from build123d import *

# Parameters (mm, degrees)
ESQUISSE1_R        = 1.5
BOSS_EXTRU_2_DEPTH = 6


with BuildPart() as part:
    # Esquisse1 → Boss.-Extru.2 (new body)
    with BuildSketch(Plane.XY):
        with BuildLine():
            Line((-4.997277712, 16.248914286), (-3.997277712, 21.633810827))
            ThreePointArc((-3.997277712, 21.633810827), (0.002768431, 21.999999826), (4.002722288, 21.632804124))
            Line((4.002722288, 21.632804124), (5.002722288, 16.247238834))
            ThreePointArc((5.002722288, 16.247238834), (8.502466554, 14.721007523), (11.573333699, 12.452226592))
            Line((11.573333699, 12.452226592), (16.7367909, 14.278649458))
            ThreePointArc((16.7367909, 14.278649458), (19.053942948, 10.997602381), (20.735919071, 7.349942877))
            Line((20.735919071, 7.349942877), (16.571882715, 3.791134828))
            ThreePointArc((16.571882715, 3.791134828), (16.999999761, -0.002848269), (16.570611412, -3.796687694))
            Line((16.570611412, -3.796687694), (20.734068613, -7.355161368))
            ThreePointArc((20.734068613, -7.355161368), (19.051174517, -11.002397445), (16.733196783, -14.282861248))
            Line((16.733196783, -14.282861248), (11.569160427, -12.456104006))
            ThreePointArc((11.569160427, -12.456104006), (8.497533208, -14.723855792), (4.997277712, -16.248914286))
            Line((4.997277712, -16.248914286), (3.997277712, -21.633810827))
            ThreePointArc((3.997277712, -21.633810827), (-0.002768431, -21.999999826), (-4.002722288, -21.632804124))
            Line((-4.002722288, -21.632804124), (-5.002722288, -16.247238834))
            ThreePointArc((-5.002722288, -16.247238834), (-8.502466554, -14.721007523), (-11.573333699, -12.452226592))
            Line((-11.573333699, -12.452226592), (-16.7367909, -14.278649458))
            ThreePointArc((-16.7367909, -14.278649458), (-19.053942948, -10.997602381), (-20.735919071, -7.349942877))
            Line((-20.735919071, -7.349942877), (-16.571882715, -3.791134828))
            ThreePointArc((-16.571882715, -3.791134828), (-16.999999761, 0.002848269), (-16.570611412, 3.796687694))
            Line((-16.570611412, 3.796687694), (-20.734068613, 7.355161368))
            ThreePointArc((-20.734068613, 7.355161368), (-19.051174517, 11.002397445), (-16.733196783, 14.282861248))
            Line((-16.733196783, 14.282861248), (-11.569160427, 12.456104006))
            ThreePointArc((-11.569160427, 12.456104006), (-8.497533208, 14.723855792), (-4.997277712, 16.248914286))
        make_face()
        with Locations((0, 14)):
            Circle(ESQUISSE1_R, mode=Mode.SUBTRACT)
        with Locations((12.124355653, -7)):
            Circle(ESQUISSE1_R, mode=Mode.SUBTRACT)
        with Locations((-12.124355653, -7)):
            Circle(ESQUISSE1_R, mode=Mode.SUBTRACT)
        with BuildLine():
            ThreePointArc((-2.411034891, 11.820685714), (0, 10.75), (2.411034891, 11.820685714))
            ThreePointArc((2.411034891, 11.820685714), (3.975330286, 12.779130538), (5.80943088, 12.737759334))
            ThreePointArc((5.80943088, 12.737759334), (11.865562564, 7.430237213), (13.995977593, -0.335575935))
            ThreePointArc((13.995977593, -0.335575935), (13.382779595, -2.564868949), (11.442531564, -3.822325392))
            ThreePointArc((11.442531564, -3.822325392), (9.309773091, -5.375), (9.031496673, -7.998360322))
            ThreePointArc((9.031496673, -7.998360322), (9.079386541, -9.832302285), (8.126507731, -11.399994391))
            ThreePointArc((8.126507731, -11.399994391), (0.5019929, -13.990997217), (-7.288606081, -11.953084179))
            ThreePointArc((-7.288606081, -11.953084179), (-8.912631465, -10.307392628), (-9.031496673, -7.998360322))
            ThreePointArc((-9.031496673, -7.998360322), (-9.309773091, -5.375), (-11.442531564, -3.822325392))
            ThreePointArc((-11.442531564, -3.822325392), (-13.054716827, -2.946828253), (-13.935938611, -1.337764944))
            ThreePointArc((-13.935938611, -1.337764944), (-12.367555464, 6.560760004), (-6.707371512, 12.288660114))
            ThreePointArc((-6.707371512, 12.288660114), (-4.47014813, 12.872261577), (-2.411034891, 11.820685714))
        make_face(mode=Mode.SUBTRACT)
    extrude(amount=BOSS_EXTRU_2_DEPTH)


solid = part.part
Geometry check sheet. Reference: the model listing, model coordinates, mm. A direction names the side the tool comes from. Give positions to 0.01 mm unless a question says otherwise; leave off trailing zeros. Loops run counter-clockwise (first coordinate to the right, second up) from the corner with the lowest first, then second, coordinate; pieces in that order, holes last.
(1) Set-up check for faces 1 (the cylindrical face through (-12.4, 6.5, 3)), 2 (the flat face through (-18.62, 5.55, 2.96)), 3 (the flat face through (14.187, -13.382, 2.958)): record each of +Z, -Z, +X, -X, +Y, -Y from which the full face is reachable in a straight line by a thin tool's end or side.
From the geometry:
face 1: +Z, -Z
face 2: +Z, -Z, -X
face 3: +Z, -Z, -Y
(2) Section check D-D on y = -18. Record the cut outline in (x, z), then the cut area to 3 significant figures.
From the geometry:
outline: (-4.68, 0) - (4.67, 0) - (4.67, 6) - (-4.68, 6) - close
area: 56.1 mm2
(3) Thickness scan on L1, parallel to Y at x = 0, z = 1.75; L2, parallel to Y at x = 11.5, z = 2.35; L3, parallel to Y at x = -18, z = 5.15. Record the ranges inside material, lowest first.
From the geometry:
L1: y = -22 to -14, 10.75 to 12.5, 15.5 to 22
L2: y = -12.52 to -8.36, -5.64 to -3.81, 7.98 to 12.52
L3: y = -12.65 to -5.01, 5.02 to 12.65
(4) Section check A-A on x = 0. Record the cut outline in (y, z), then the cut area to 3 significant figures.
From the geometry:
outline: (-22, 0) - (-14, 0) - (-14, 6) - (-22, 6) - close; (10.75, 0) - (12.5, 0) - (12.5, 6) - (10.75, 6) - close; (15.5, 0) - (22, 0) - (22, 6) - (15.5, 6) - close
area: 97.5 mm2
(5) Depth check by flat-ended pin: pin 1 Ø2 at (x, z) = (14.5, 1.5) entering from +Y; pin 2 Ø1 at (x, z) = (-12.5, 2.5) entering from -Y; pin 3 Ø1.5 at (y, z) = (4.5, 2.5) entering from -X. Enter the tip coordinate at first touch or a pass-through.
From the geometry:
pin 1: stops at y = 13.84
pin 2: stops at y = -12.96
pin 3: stops at x = -18.27
(6) Release check for a two-part mould opening along Y. For faces 4 (the flat face through (4.504, -18.904, 2.958)), 5 (the flat face through (4.496, 18.978, 2.958)), 6 (the cylindrical face through (11.804, 7.527, 2.958)) record: released by +Y, released by -Y, zero draft, split by the parting line, or undercut.
From the geometry:
face 4: released by -Y
face 5: released by +Y
face 6: undercut
(7) Section check C-C on z = 3.5. Count the separate pieces of the cut face and the enclosed holes in it, then the cut area to 3 significant figures.
From the geometry:
separate pieces: 1
enclosed holes: 4
area: 599 mm2
(8) Section check B-B on y = -9.5. Record the cut outline in (x, z).
From the geometry:
outline: (-19.84, 0) - (-9.15, 0) - (-9.15, 6) - (-19.84, 6) - close; (9.15, 0) - (19.84, 0) - (19.84, 6) - (9.15, 6) - close
